For this review, take the finished solid that the model builds, in its own axes (mm). A direction names the side the tool comes from. Coordinates: 2 decimals unless noted, no trailing zeros. Loops run counter-clockwise (first coordinate to the right, second up) from the corner with the lowest first, then second, coordinate; pieces in that order, holes last. Notation, with made-up numbers: (-1.75, 55) - (31.25, 55) arc R5 cw to (31.25, 63) - close; hole circle Ø5 at (82.5, -26.5). An arc over 180 degrees is marked (long way). Answer as a JSON object with one key per item and string values. Group by question number.
Item 1: We need section C-C (x = 5). Give the boundary of the cut face in (y, z), then the cut area to 3 significant figures.
Item 2: We need section D-D (z = -0.55). Give the boundary of the cut face in (x, y), then the cut area to 3 significant figures.
Item 3: We need section A-A (y = 0). Give the boundary of the cut face in (x, z).
Item 4: Tool access review of faces 5 (the flat face through (-0.1, -4.3, 0)), 6 (the flat face through (1, -3, -1)): name each direction out of +Z, -Z, +X, -X, +Y, -Y from which nothing blocks a thin tool from reaching the whole face with its end or side.
Item 5: Clearance check with flat-ended pins moving along their axes: pin 1 (5.5 mm diameter, centred on x = 0, y = 0, fed in from +Z); pin 2 (5 mm diameter, centred on x = -5, y = -5, fed in from -Z); pin 3 (1.5 mm diameter, centred on y = -4.5, z = 0.5, fed in from -X). State where each tip first meets the part, or that it passes through.
Item 6: Mouldability with a two-part tool opening along Y and no side actions: class faces 1 (the flat face through (-2.4, -2.1, 2)), 2 (the cylindrical face through (-5.806, -3.735, 0.986)), 3 (the cylindrical face through (-6.386, 4.425, 0.986)), 4 (the cylindrical face through (-0.867, 3.905, -0.493)) as released by +Y, released by -Y, zero draft, split by the parting line, or undercut.
Item 7: To check wall thickness, follow line 1 (Y direction, x = -4, z = 1.4); line 2 (Z direction, x = -7.75, y = 1.25). State the ranges of each line that lie inside material, in increasing order.
from build123d import *

# Parameters (mm, degrees)
F0_R     = 10
F0_R_2   = 3
F1_DEPTH = 2
F3_D     = 3
F4_R     = 4
F4_R_2   = 3
F5_DEPTH = 1


with BuildPart() as f1:
    # F0 (on Top) → F1 (new body)
    with BuildSketch(Plane.XY):
        Circle(F0_R)
        Circle(F0_R_2, mode=Mode.SUBTRACT)
    extrude(amount=F1_DEPTH)

    # F3 (through all)
    with Locations(Plane.XY.offset(2)):
        with Locations((-5, 5), (5, 5), (5, -5), (-5, -5)):
            Hole(F3_D / 2)

    # F4 (on face) → F5 (join)
    with BuildSketch(Plane(origin=(0, 0, 0), x_dir=(1, 0, 0), z_dir=(0, 0, -1))):
        Circle(F4_R)
        Circle(F4_R_2, mode=Mode.SUBTRACT)
    extrude(amount=F5_DEPTH)


solid = f1.part
Check sheet entries:
{
 "1": {"outline": "(-8.66, 0) - (-6.5, 0) - (-6.5, 2) - (-8.66, 2) - close; (-3.5, 0) - (3.5, 0) - (3.5, 2) - (-3.5, 2) - close; (6.5, 0) - (8.66, 0) - (8.66, 2) - (6.5, 2) - close", "area": "22.6 mm2"},
 "2": {"outline": "circle Ø8 at (0, 0); hole circle Ø6 at (0, 0)", "area": "22.0 mm2"},
 "3": {"outline": "(-10, 0) - (-4, 0) - (-4, -1) - (-3, -1) - (-3, 2) - (-10, 2) - close; (3, -1) - (4, -1) - (4, 0) - (10, 0) - (10, 2) - (3, 2) - close"},
 "4": {"face 5": "-Z", "face 6": "-Z, +X, -X, +Y, -Y"},
 "5": {"pin 1": "passes through", "pin 2": "stops at z = 0", "pin 3": "stops at x = -9.27"},
 "6": {"face 1": "zero draft", "face 2": "undercut", "face 3": "undercut", "face 4": "split by the parting line"},
 "7": {"line 1": "y = -9.17 to -6.12, -3.88 to 3.88, 6.12 to 9.17", "line 2": "z = 0 to 2"}
}
